Build history of the part. All positions in model axes, mm. A direction names the side the tool comes from. Round coordinates to 2 decimals unless told otherwise and drop trailing zeros. Write each loop counter-clockwise with the first axis right and the second up, starting at its lowest first coordinate (ties: lowest second). Pieces come first, ordered by that corner, then holes.
from build123d import *

# Parameters (mm, degrees)
SKETCH1_W             = 127
SKETCH1_H             = 25.4
BOSS_EXTRUDE1_DEPTH   = 6.35
F_8_CLEARANCE_HOLE2_D = 4.4958
LPATTERN1_COUNT       = 2
LPATTERN1_PITCH       = 139.7
LPATTERN1_COUNT_DIR2  = 2
LPATTERN1_PITCH_DIR2  = 139.7


with BuildPart() as part:
    # Sketch1 → Boss-Extrude1 (new body)
    with BuildSketch(Plane.XY):
        Polygon((-163.974683544, 121.551475626), (-163.974683544, 83.451475626), (-316.374683544, 83.451475626), (-316.374683544, 121.551475626), (-316.374683544, 235.851475626), (-163.974683544, 235.851475626), align=None)
        with Locations((-240.174683544, 108.851475626)):
            Rectangle(SKETCH1_W, SKETCH1_H, mode=Mode.SUBTRACT)
        with BuildLine():
            Line((-303.674683544, 121.551475626), (-303.674683544, 115.201475626))
            ThreePointArc((-303.674683544, 115.201475626), (-301.814811605, 119.691603686), (-297.324683544, 121.551475626))
            Line((-297.324683544, 121.551475626), (-303.674683544, 121.551475626))
        make_face()
        with BuildLine():
            Line((-303.674683544, 102.501475626), (-303.674683544, 96.151475626))
            Line((-303.674683544, 96.151475626), (-297.324683544, 96.151475626))
            ThreePointArc((-297.324683544, 96.151475626), (-301.814811605, 98.011347565), (-303.674683544, 102.501475626))
        make_face()
        with BuildLine():
            ThreePointArc((-183.024683544, 121.551475626), (-178.534555484, 119.691603686), (-176.674683544, 115.201475626))
            Line((-176.674683544, 115.201475626), (-176.674683544, 121.551475626))
            Line((-176.674683544, 121.551475626), (-183.024683544, 121.551475626))
        make_face()
        with BuildLine():
            ThreePointArc((-176.674683544, 102.501475626), (-178.534555484, 98.011347565), (-183.024683544, 96.151475626))
            Line((-183.024683544, 96.151475626), (-176.674683544, 96.151475626))
            Line((-176.674683544, 96.151475626), (-176.674683544, 102.501475626))
        make_face()
    extrude(amount=BOSS_EXTRUDE1_DEPTH)

    # #8 Clearance Hole2 (through all)
    with Locations(Plane.XY.offset(6.35)):
        with Locations((-310.051516204, 229.517938536)):
            f_8_clearance_hole2 = Hole(F_8_CLEARANCE_HOLE2_D / 2)

    # LPattern1: 8 Clearance Hole2 2 × 2
    with Locations(*[(j * LPATTERN1_PITCH_DIR2, -i * LPATTERN1_PITCH, 0) for i in range(LPATTERN1_COUNT) for j in range(LPATTERN1_COUNT_DIR2) if (i, j) != (0, 0)]):
        add(f_8_clearance_hole2, mode=Mode.SUBTRACT)


solid = part.part
1) Wall check: L1, parallel to Y at x = -259.5, z = 4.5; L2, parallel to Y at x = -171.5, z = 0.5; L3, parallel to X at y = 115, z = 3.25. Give the ranges that are in metal, low to high.
Results:
L1: y = 83.45 to 96.15, 121.55 to 235.85
L2: y = 83.45 to 87.89, 91.75 to 227.59, 231.45 to 235.85
L3: x = -316.37 to -303.67, -176.67 to -163.97
2) Slice it at A-A (x = -266.5). Write the cut outline in (y, z).
Results:
outline: (83.45, 0) - (96.15, 0) - (96.15, 6.35) - (83.45, 6.35) - close; (121.55, 0) - (235.85, 0) - (235.85, 6.35) - (121.55, 6.35) - close
3) Slice it at B-B (y = 100). Write the cut outline in (x, z).
Results:
outline: (-316.37, 0) - (-303.16, 0) - (-303.16, 6.35) - (-316.37, 6.35) - close; (-177.19, 0) - (-163.97, 0) - (-163.97, 6.35) - (-177.19, 6.35) - close
4) Mould opens along Y. For faces 3 (the flat face through (-163.975, 159, 3)), 4 (the cylindrical face through (-301.765, 97.962, 3.131)), 5 (the flat face through (-241, 235.851, 3)) say: released by +Y, released by -Y, zero draft, split by the parting line, or undercut.
Results:
face 3: zero draft
face 4: undercut
face 5: released by +Y
5) Which spindle directions (+Z, -Z, +X, -X, +Y, -Y) get a long thin tool onto all of the face, cutting with end or side? Do faces 1 (the flat face through (-241, 121.551, 3)), 2 (the flat face through (-239, 83.451, 3)). Say none if no direction does.
Results:
face 1: +Z, -Z
face 2: +Z, -Z, +X, -X, -Y
6) Slice it at C-C (z = 2). Write the cut outline in (x, y), plus the area to 3 significant figures.
Results:
outline: (-316.37, 83.45) - (-163.97, 83.45) - (-163.97, 235.85) - (-316.37, 235.85) - close; hole circle Ø4.5 at (-310.05, 89.82); hole circle Ø4.5 at (-310.05, 229.52); hole (-303.67, 102.5) arc R6.35 ccw to (-297.32, 96.15) - (-183.02, 96.15) arc R6.35 ccw to (-176.67, 102.5) - (-176.67, 115.2) arc R6.35 ccw to (-183.02, 121.55) - (-297.32, 121.55) arc R6.35 ccw to (-303.67, 115.2) - close; hole circle Ø4.5 at (-170.35, 89.82); hole circle Ø4.5 at (-170.35, 229.52)
area: 20,000 mm2
